```python
from build123d import *

# Parameters (mm, degrees)
SKETCH_1_R          = 5
SKETCH_1_R_2        = 3
EXTRUDE_1_DEPTH     = 9
SKETCH_2_R          = 3.75
CUT_EXTRUDE_1_DEPTH = 2
SKETCH_3_R          = 2.9
EXTRUDE_2_DEPTH     = 3
FILLET_1_R          = 2
SKETCH_4_R          = 2.9
EXTRUDE_3_DEPTH     = 10
FILLET_2_R          = 2.9
FILLET_3_R          = 3


with BuildPart() as part:
    # 스케치1 → 보스-돌출1 (new body)
    # profile 1 of 5: a face of its own
    with BuildSketch(Plane.XY):
        with BuildLine():
            Line((8.866410343, 21.94338903), (4.384187039, 21.94338903))
            Line((4.384187039, 21.94338903), (2.987768149, 19.65002342))
            Line((2.987768149, 19.65002342), (2.987768149, 17.661246793))
            Line((2.987768149, 17.661246793), (2.987768149, 9.70876495))
            Line((2.987768149, 9.70876495), (-3.184671245, 3.854590647))
            ThreePointArc((-3.184671245, 3.854590647), (2.13033375, 4.523458645), (5, 0))
            ThreePointArc((5, 0), (0, -5), (-5, 0))
            Line((-5, 0), (-5, -10.071407464))
            Line((-5, -10.071407464), (-16.264805165, -9.728236855))
            Line((-16.264805165, -9.728236855), (-17.766639728, -13.42657959))
            Line((-17.766639728, -13.42657959), (-19.940502755, -13.22881584))
            ThreePointArc((-19.940502755, -13.22881584), (-21.568981751, -13.840235901), (-22.102673306, -15.49581787))
            ThreePointArc((-22.102673306, -15.49581787), (-21.54079944, -16.765444299), (-20.287735083, -17.363343312))
            Line((-20.287735083, -17.363343312), (-13.716958703, -17.9611093))
            ThreePointArc((-13.716958703, -17.9611093), (-10.295562947, -19.77999502), (-9.201017746, -23.497018692))
            Line((-9.201017746, -23.497018692), (-13.218080179, -30.193463728))
            ThreePointArc((-13.218080179, -30.193463728), (-13.817495958, -30.9099569), (-14.608237914, -31.407338947))
            Line((-14.608237914, -31.407338947), (-15.296022277, -31.702310231))
            ThreePointArc((-15.296022277, -31.702310231), (-15.622210934, -31.927735325), (-15.835150792, -32.262208238))
            ThreePointArc((-15.835150792, -32.262208238), (-16.003126851, -45.501568691), (-10.133257231, -57.36974091))
            ThreePointArc((-10.133257231, -57.36974091), (-7.618845179, -57.635707988), (-7.276099317, -55.130606848))
            ThreePointArc((-7.276099317, -55.130606848), (-11.022489697, -44.432594757), (-8.133553397, -33.471894478))
            ThreePointArc((-8.133553397, -33.471894478), (-7.245000489, -32.901805175), (-6.337557558, -32.362291125))
            ThreePointArc((-6.337557558, -32.362291125), (-5.290911527, -31.673468731), (-4.338619501, -30.85916897))
            Line((-4.338619501, -30.85916897), (6.238088337, -20.600518625))
            Line((6.238088337, -20.600518625), (8.3701186, -14.978169718))
            ThreePointArc((8.3701186, -14.978169718), (8.662275884, -14.729272874), (8.69193724, -14.346616734))
            ThreePointArc((8.69193724, -14.346616734), (8.365752146, -12.021808556), (8.866410343, -9.728236855))
            Line((8.866410343, -9.728236855), (8.866410343, 21.94338903))
        make_face()
    # profile 2 of 5: a face of its own
    with BuildSketch(Plane.XY):
        Circle(SKETCH_1_R)
        Circle(SKETCH_1_R_2, mode=Mode.SUBTRACT)
    # profile 3 of 5: a face of its own
    with BuildSketch(Plane.XY):
        with BuildLine():
            ThreePointArc((5, 0), (2.13033375, 4.523458645), (-3.184671245, 3.854590647))
            ThreePointArc((-3.184671245, 3.854590647), (-4.523458645, 2.13033375), (-5, 0))
            ThreePointArc((-5, 0), (0, -5), (5, 0))
        make_face()
        Circle(SKETCH_1_R_2, mode=Mode.SUBTRACT)
    # profile 4 of 5: a face of its own
    with BuildSketch(Plane.XY):
        Polygon((8.866410343, 25.078081763), (7.518879772, 25.078081763), (4.384187039, 21.94338903), (8.866410343, 21.94338903), align=None)
    # profile 5 of 5: a face of its own
    with BuildSketch(Plane.XY):
        with BuildLine():
            Line((8.866410343, 21.94338903), (4.384187039, 21.94338903))
            Line((4.384187039, 21.94338903), (2.987768149, 19.65002342))
            Line((2.987768149, 19.65002342), (2.987768149, 17.661246793))
            Line((2.987768149, 17.661246793), (2.987768149, 9.70876495))
            Line((2.987768149, 9.70876495), (-3.184671245, 3.854590647))
            ThreePointArc((-3.184671245, 3.854590647), (2.13033375, 4.523458645), (5, 0))
            ThreePointArc((5, 0), (0, -5), (-5, 0))
            Line((-5, 0), (-5, -10.071407464))
            Line((-5, -10.071407464), (-16.264805165, -9.728236855))
            Line((-16.264805165, -9.728236855), (-17.766639728, -13.42657959))
            Line((-17.766639728, -13.42657959), (-19.940502755, -13.22881584))
            ThreePointArc((-19.940502755, -13.22881584), (-21.568981751, -13.840235901), (-22.102673306, -15.49581787))
            ThreePointArc((-22.102673306, -15.49581787), (-21.54079944, -16.765444299), (-20.287735083, -17.363343312))
            Line((-20.287735083, -17.363343312), (-13.716958703, -17.9611093))
            ThreePointArc((-13.716958703, -17.9611093), (-10.295562947, -19.77999502), (-9.201017746, -23.497018692))
            Line((-9.201017746, -23.497018692), (-13.218080179, -30.193463728))
            ThreePointArc((-13.218080179, -30.193463728), (-13.817495958, -30.9099569), (-14.608237914, -31.407338947))
            Line((-14.608237914, -31.407338947), (-15.296022277, -31.702310231))
            ThreePointArc((-15.296022277, -31.702310231), (-15.622210934, -31.927735325), (-15.835150792, -32.262208238))
            ThreePointArc((-15.835150792, -32.262208238), (-16.003126851, -45.501568691), (-10.133257231, -57.36974091))
            ThreePointArc((-10.133257231, -57.36974091), (-7.618845179, -57.635707988), (-7.276099317, -55.130606848))
            ThreePointArc((-7.276099317, -55.130606848), (-11.022489697, -44.432594757), (-8.133553397, -33.471894478))
            ThreePointArc((-8.133553397, -33.471894478), (-7.245000489, -32.901805175), (-6.337557558, -32.362291125))
            ThreePointArc((-6.337557558, -32.362291125), (-5.290911527, -31.673468731), (-4.338619501, -30.85916897))
            Line((-4.338619501, -30.85916897), (6.238088337, -20.600518625))
            Line((6.238088337, -20.600518625), (8.3701186, -14.978169718))
            ThreePointArc((8.3701186, -14.978169718), (8.662275884, -14.729272874), (8.69193724, -14.346616734))
            ThreePointArc((8.69193724, -14.346616734), (8.365752146, -12.021808556), (8.866410343, -9.728236855))
            Line((8.866410343, -9.728236855), (8.866410343, 21.94338903))
        make_face()
    extrude(amount=EXTRUDE_1_DEPTH)

    # 스케치2 → 컷-돌출1 (cut)
    with BuildSketch(Plane(origin=(8.866410343, 0, 0), x_dir=(0, 0, -1), z_dir=(1, 0, 0))):
        with Locations(Location((-4.5, 15.078081763, 0), (0, 0, 90))):
            Circle(SKETCH_2_R)
    extrude(amount=-CUT_EXTRUDE_1_DEPTH, mode=Mode.SUBTRACT)

    # 스케치3 → 보스-돌출2 (add)
    with BuildSketch(Plane(origin=(6.866410343, 0, 0), x_dir=(0, 0, -1), z_dir=(1, 0, 0))):
        with Locations(Location((-4.5, 15.078081763, 0), (0, 0, 90))):
            Circle(SKETCH_3_R)
    extrude(amount=EXTRUDE_2_DEPTH)

    # 필렛1
    fillet_1_edges = [part.edges().sort_by_distance(p)[0] for p in [
        (9.866410343, 12.178081763, 4.5),
    ]]
    fillet(fillet_1_edges, radius=FILLET_1_R)

    # 스케치4 → 보스-돌출3 (add)
    with BuildSketch(Plane(origin=(-1.357268469, -14.919396185, 0), x_dir=(0.995887428286197, -0.09059928355955607, 0), z_dir=(0.09059928355955607, 0.995887428286197, 0))):
        with Locations(Location((-11.65777439, -4.5, 0), (0, 0, 180))):
            Circle(SKETCH_4_R)
    extrude(amount=EXTRUDE_3_DEPTH)

    # 필렛2
    fillet_2_edges = [part.edges().sort_by_distance(p)[0] for p in [
        (-9.173033049, -4.167073817, 4.5),
    ]]
    fillet(fillet_2_edges, radius=FILLET_2_R)

    # 필렛3
    fillet_3_edges = [part.edges().sort_by_distance(p)[0] for p in [
        (-5, -10.071407464, 4.5),
    ]]
    fillet(fillet_3_edges, radius=FILLET_3_R)


solid = part.part
```
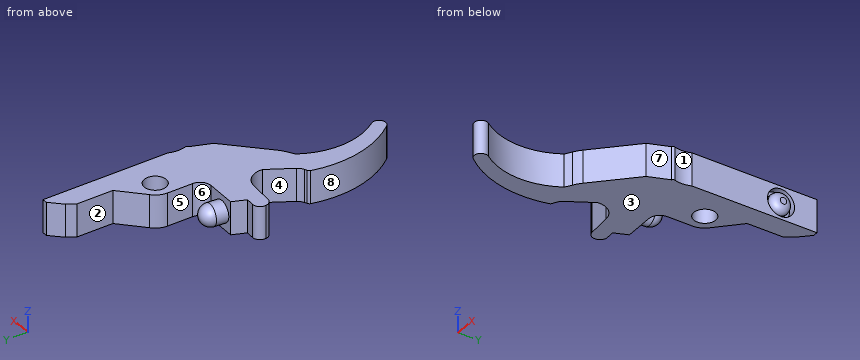
Input: part model. Units: mm. Frame: model coordinates. Face numbers are marked on the shaded views. A direction names the side the tool comes from. Give positions to 0.01 mm unless a question says otherwise; leave off trailing zeros. Order: outer loops, then holes, each group sorted by start corner. A loop starts at its lowest first (then second) coordinate and runs counter-clockwise, first axis right, second up. Notation, with made-up numbers: M -20,-10.75 L 25,-10.75 A19 cw 25,-4.75 Z; hole C 53,10.5 d6. An arc over 180 degrees is marked long. One line per question, with ' | ' between items.
1) Contact query for flat-ended pins moving along their axis: P1, Ø2, axis at y = -3.5, z = 3, coming from the -X side; P2, Ø3, axis at x = -18.5, z = 1.5, coming from the +Y side; P3, Ø3, axis at x = -18, y = -44, coming from the +Z side; P4, Ø5, axis at y = -48, z = 2.5, coming from the -X side. Output: stop coordinate, or through.
Filled in:
P1: stops at x = -13.57 | P2: stops at y = -11.54 | P3: passes through | P4: stops at x = -16
2) Section A-A on y = 8. Output: boundary loops of the cut face in (x, z).
Filled in:
outline: M 1.19,0 L 8.87,0 L 8.87,9 L 1.19,9 Z
3) Draft query along Y for the marked faces 6, 7 and 8. Return one class per face: pulls with the +Y half, pulls with the -Y half, needs draft (parallel to the pull), parting line crosses it, or undercut.
Filled in:
face 6: pulls with the +Y half | face 7: pulls with the -Y half | face 8: undercut
4) Access query for the marked faces 1, 2, 3, 4 and 5. Directions: +Z, -Z, +X, -X, +Y, -Y. A direction counts if a zero-diameter tool reaches every point of the face in a straight line with its end or side. Return the directions, or none.
Filled in:
face 1: +Z, -Z, +X | face 2: +Z, -Z, -X, +Y | face 3: -Z, +X, -X, +Y, -Y | face 4: +Z, -Z, -X | face 5: +Z, -Z, +Y
5) Ray query, L1, parallel to Y at x = 2, z = 6; L2, parallel to X at y = -6.5, z = 3.5; L3, parallel to X at y = 6, z = 2.75. Return the intervals inside material, ascending.
Filled in:
L1: y = -24.71 to -2.24, 2.24 to 8.77 | L2: x = -15.03 to -9.62, -5 to 8.87 | L3: x = -0.92 to 8.87
